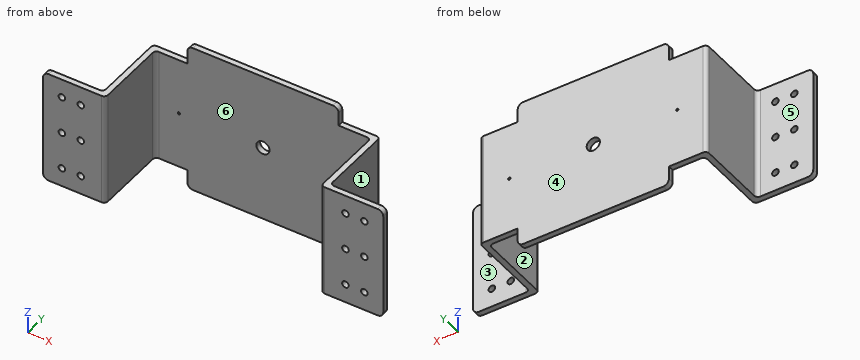
```python
from build123d import *

# Parameters (mm, degrees)
SKETCH_1_W                  = 120
SKETCH_1_H                  = 60
EXTRUDE_1_DEPTH             = 3
SKETCH_2_W                  = 3
SKETCH_2_H                  = 60
EXTRUDE_2_DEPTH             = 40
SKETCH_3_W                  = 60
SKETCH_3_H                  = 3
EXTRUDE_3_DEPTH             = 30
SKETCH_4_R                  = 1.75
CUT_EXTRUDE_1_DEPTH         = 3
PATTERN_LINEAR_1_COUNT      = 3
PATTERN_LINEAR_1_PITCH      = 20
PATTERN_LINEAR_1_COUNT_DIR2 = 2
PATTERN_LINEAR_1_PITCH_DIR2 = 10
MIRROR_1_COPY_1_SKETCH_R    = 1.75
MIRROR_1_COPY_1_DEPTH       = 3
MIRROR_1_COPY_2_SKETCH_R    = 1.75
MIRROR_1_COPY_2_DEPTH       = 3
MIRROR_1_COPY_3_SKETCH_R    = 1.75
MIRROR_1_COPY_3_DEPTH       = 3
MIRROR_1_COPY_4_SKETCH_R    = 1.75
MIRROR_1_COPY_4_DEPTH       = 3
MIRROR_1_COPY_5_SKETCH_R    = 1.75
MIRROR_1_COPY_5_DEPTH       = 3
SKETCH_5_R                  = 3.5
CUT_EXTRUDE_2_DEPTH         = 3
SKETCH_6_R                  = 0.5
CUT_EXTRUDE_3_DEPTH         = 3
SKETCH_7_W                  = 80
SKETCH_7_H                  = 10
EXTRUDE_4_DEPTH             = 3
FILLET_1_R                  = 3
FILLET_2_R                  = 3
HOLE_WIZARD_M1_6_1_D        = 1.25
FILLET_3_R                  = 2
FILLET_4_R                  = 2
FILLET_5_R                  = 3


with BuildPart() as part:
    # 草图1 → 凸台-拉伸1 (new body)
    with BuildSketch(Plane(origin=(0, 0, 0), x_dir=(1, 0, 0), z_dir=(0, 1, 0))):
        Rectangle(SKETCH_1_W, SKETCH_1_H)
    extrude(amount=EXTRUDE_1_DEPTH)

    # 草图2 → 凸台-拉伸2 (add)
    with BuildSketch(Plane.XZ):
        with Locations((-58.5, 0)):
            Rectangle(SKETCH_2_W, SKETCH_2_H)
    extrude_2 = extrude(amount=EXTRUDE_2_DEPTH)

    # 草图3 → 凸台-拉伸3 (add)
    with BuildSketch(Plane.ZY.offset(60)):
        with Locations((0, -38.5)):
            Rectangle(SKETCH_3_W, SKETCH_3_H)
    extrude_3 = extrude(amount=EXTRUDE_3_DEPTH)

    # 草图4 → 切除-拉伸1 (cut)
    with BuildSketch(Plane(origin=(0, -37, 0), x_dir=(1, 0, 0), z_dir=(0, 1, 0))):
        with Locations(Location((-70, -20, 0), (0, 0, 270))):
            Circle(SKETCH_4_R)
    cut_extrude_1 = extrude(amount=-CUT_EXTRUDE_1_DEPTH, mode=Mode.SUBTRACT)

    # 阵列(线性)1: Cut-Extrude 1 3 × 2
    with Locations(*[(-j * PATTERN_LINEAR_1_PITCH_DIR2, 0, -i * PATTERN_LINEAR_1_PITCH) for i in range(PATTERN_LINEAR_1_COUNT) for j in range(PATTERN_LINEAR_1_COUNT_DIR2) if (i, j) != (0, 0)]):
        add(cut_extrude_1, mode=Mode.SUBTRACT)

    # 镜向1: 凸台-拉伸2, 凸台-拉伸3, 切除-拉伸1 across plane
    add(extrude_2.mirror(Plane(origin=(0, 0, 0), x_dir=(0, 0, 1), z_dir=(1, 0, 0))))
    add(extrude_3.mirror(Plane(origin=(0, 0, 0), x_dir=(0, 0, 1), z_dir=(1, 0, 0))))
    add(cut_extrude_1.mirror(Plane(origin=(0, 0, 0), x_dir=(0, 0, 1), z_dir=(1, 0, 0))), mode=Mode.SUBTRACT)

    # 镜向1 copy 1 sketch → 镜向1 copy 1 (cut)
    with BuildSketch(Plane(origin=(10, -37, 0), x_dir=(-1, 0, 0), z_dir=(0, 1, 0))):
        with Locations((-70, 20)):
            Circle(MIRROR_1_COPY_1_SKETCH_R)
    extrude(amount=-MIRROR_1_COPY_1_DEPTH, mode=Mode.SUBTRACT)

    # 镜向1 copy 2 sketch → 镜向1 copy 2 (cut)
    with BuildSketch(Plane(origin=(0, -37, -20), x_dir=(-1, 0, 0), z_dir=(0, 1, 0))):
        with Locations((-70, 20)):
            Circle(MIRROR_1_COPY_2_SKETCH_R)
    extrude(amount=-MIRROR_1_COPY_2_DEPTH, mode=Mode.SUBTRACT)

    # 镜向1 copy 3 sketch → 镜向1 copy 3 (cut)
    with BuildSketch(Plane(origin=(10, -37, -20), x_dir=(-1, 0, 0), z_dir=(0, 1, 0))):
        with Locations((-70, 20)):
            Circle(MIRROR_1_COPY_3_SKETCH_R)
    extrude(amount=-MIRROR_1_COPY_3_DEPTH, mode=Mode.SUBTRACT)

    # 镜向1 copy 4 sketch → 镜向1 copy 4 (cut)
    with BuildSketch(Plane(origin=(0, -37, -40), x_dir=(-1, 0, 0), z_dir=(0, 1, 0))):
        with Locations((-70, 20)):
            Circle(MIRROR_1_COPY_4_SKETCH_R)
    extrude(amount=-MIRROR_1_COPY_4_DEPTH, mode=Mode.SUBTRACT)

    # 镜向1 copy 5 sketch → 镜向1 copy 5 (cut)
    with BuildSketch(Plane(origin=(10, -37, -40), x_dir=(-1, 0, 0), z_dir=(0, 1, 0))):
        with Locations((-70, 20)):
            Circle(MIRROR_1_COPY_5_SKETCH_R)
    extrude(amount=-MIRROR_1_COPY_5_DEPTH, mode=Mode.SUBTRACT)

    # 草图5 → 切除-拉伸2 (cut)
    with BuildSketch(Plane(origin=(0, 3, 0), x_dir=(1, 0, 0), z_dir=(0, 1, 0))):
        with Locations(Location((0, 0, 0), (0, 0, 270))):
            Circle(SKETCH_5_R)
    extrude(amount=-CUT_EXTRUDE_2_DEPTH, mode=Mode.SUBTRACT)

    # 草图6 → 切除-拉伸3 (cut)
    with BuildSketch(Plane(origin=(0, 3, 0), x_dir=(1, 0, 0), z_dir=(0, 1, 0))):
        with Locations(Location((44.45, 0, 0), (0, 0, 270))):
            Circle(SKETCH_6_R)
    cut_extrude_3 = extrude(amount=-CUT_EXTRUDE_3_DEPTH, mode=Mode.SUBTRACT)

    # 镜向2: 切除-拉伸3 across plane
    add(cut_extrude_3.mirror(Plane(origin=(0, 0, 0), x_dir=(0, 0, 1), z_dir=(1, 0, 0))), mode=Mode.SUBTRACT)

    # 草图7 → 凸台-拉伸4 (add)
    with BuildSketch(Plane(origin=(0, 3, 0), x_dir=(1, 0, 0), z_dir=(0, 1, 0))):
        with Locations((0, 35)):
            Rectangle(SKETCH_7_W, SKETCH_7_H)
    extrude_4 = extrude(amount=-EXTRUDE_4_DEPTH)

    # 镜向3: 凸台-拉伸4 across plane
    add(extrude_4.mirror(Plane.XY))

    # 圆角1
    fillet_1_edges = [part.edges().sort_by_distance(p)[0] for p in [
        (-40, 1.5, 40),
    ]]
    fillet(fillet_1_edges, radius=FILLET_1_R)

    # 圆角2
    fillet_2_edges = [part.edges().sort_by_distance(p)[0] for p in [
        (-40, 1.5, -40),
        (40, 1.5, -40),
        (40, 1.5, 40),
    ]]
    fillet(fillet_2_edges, radius=FILLET_2_R)

    # M1.6 螺纹孔1 (through all)
    with Locations(Plane(origin=(0, 3, 0), x_dir=(1, 0, 0), z_dir=(0, 1, 0))):
        with Locations((44.45, 0), (-44.45, 0)):
            Hole(HOLE_WIZARD_M1_6_1_D / 2)

    # 圆角3
    fillet_3_edges = [part.edges().sort_by_distance(p)[0] for p in [
        (-57, 0, 0),
        (-60, 3, 0),
    ]]
    fillet(fillet_3_edges, radius=FILLET_3_R)

    # 圆角4
    fillet_4_edges = [part.edges().sort_by_distance(p)[0] for p in [
        (60, 3, 0),
        (-57, -40, 0),
        (-60, -37, 0),
        (57, -40, 0),
        (57, 0, 0),
        (60, -37, 0),
    ]]
    fillet(fillet_4_edges, radius=FILLET_4_R)

    # 圆角5
    fillet_5_edges = [part.edges().sort_by_distance(p)[0] for p in [
        (-90, -38.5, -30),
        (-90, -38.5, 30),
        (90, -38.5, -30),
        (90, -38.5, 30),
    ]]
    fillet(fillet_5_edges, radius=FILLET_5_R)


solid = part.part
```
Part model, mm, in its own coordinate system. Face numbers are marked on the shaded views. A direction names the side the tool comes from. Give positions to 0.01 mm unless a question says otherwise; leave off trailing zeros. Write each loop counter-clockwise with the first axis right and the second up, starting at its lowest first coordinate (ties: lowest second). Pieces come first, ordered by that corner, then holes. Notation, with made-up numbers: (52.5, 68) -> (83.5, 68) arc R13 ccw to (83.5, 85) -> close; hole circle Ø7 at (50.25, 8). An arc over 180 degrees is marked (long way). Put each result on its own line as item: value. Start each with the question number.
Item 1: Cut at D-D (x = -80). List the corners of the cut face in (y, z), then the cut area to 4 significant figures.
Item 2: Wall check: L1, parallel to Z at x = -70, y = -38.75; L2, parallel to Z at x = -44.45, y = 1.9 (3 decimals); L3, parallel to X at y = -23.5, z = 11.5. Give the ranges that are in metal, low to high. Write a range as [from, to].
Item 3: Cut at A-A (x = 0). List the corners of the cut face in (y, z).
Item 4: Cut at B-B (y = -29). List the corners of the cut face in (x, z), then the cut area to 3 significant figures.
Item 5: Cut at C-C (z = -16). List the corners of the cut face in (x, y), then the cut area to 3 significant figures.
Item 6: Which spindle directions (+Z, -Z, +X, -X, +Y, -Y) get a long thin tool onto all of the face, cutting with end or side? Do the marked faces 4, 5 and 6. Say none if no direction does.
Item 7: Pin check, flat tips, straight feed: pin 1 Ø5 at (x, y) = (-50, -4.5) entering from +Z; pin 2 Ø1.4 at (x, z) = (44.45, 0) entering from -Y; pin 3 Ø4.5 at (x, z) = (-80, 20) entering from -Y; pin 4 Ø3 at (y, z) = (-32.5, -7) entering from -X. Stop position of each tip, or through.
Item 8: Pull direction X, two halves, no side cores. Call the marked faces 1, 2 and 3: pulls with the +X half, pulls with the -X half, needs draft (parallel to the pull), parting line crosses it, or undercut.
Answer list:
1. outline: (-40, -30) -> (-37, -30) -> (-37, -21.75) -> (-40, -21.75) -> close; (-40, -18.25) -> (-37, -18.25) -> (-37, -1.75) -> (-40, -1.75) -> close; (-40, 1.75) -> (-37, 1.75) -> (-37, 18.25) -> (-40, 18.25) -> close; (-40, 21.75) -> (-37, 21.75) -> (-37, 30) -> (-40, 30) -> close
1. area: 148.5 mm2
2. L1: z = [-30, -21.75], [-18.25, -1.75], [1.75, 18.25], [21.75, 30]
2. L2: z = [-30, -0.625], [0.625, 30]
2. L3: x = [-60, -57], [57, 60]
3. outline: (0, -40) -> (3, -40) -> (3, -3.5) -> (0, -3.5) -> close; (0, 3.5) -> (3, 3.5) -> (3, 40) -> (0, 40) -> close
4. outline: (-60, -30) -> (-57, -30) -> (-57, 30) -> (-60, 30) -> close; (57, -30) -> (60, -30) -> (60, 30) -> (57, 30) -> close
4. area: 360 mm2
5. outline: (-90, -40) -> (-59, -40) arc R2 ccw to (-57, -38) -> (-57, -2) arc R2 cw to (-55, 0) -> (55, 0) arc R2 cw to (57, -2) -> (57, -38) arc R2 ccw to (59, -40) -> (90, -40) -> (90, -37) -> (62, -37) arc R2 cw to (60, -35) -> (60, 1) arc R2 ccw to (58, 3) -> (-58, 3) arc R2 ccw to (-60, 1) -> (-60, -35) arc R2 cw to (-62, -37) -> (-90, -37) -> close
5. area: 780 mm2
6. face 4: +Z, -Z, +X, -X, +Y
6. face 5: +Z, -Z, -X, +Y
6. face 6: +Z, -Z, -Y
7. pin 1: passes through
7. pin 2: stops at y = 0
7. pin 3: stops at y = -40
7. pin 4: stops at x = -60
8. face 1: pulls with the +X half
8. face 2: undercut
8. face 3: needs draft
